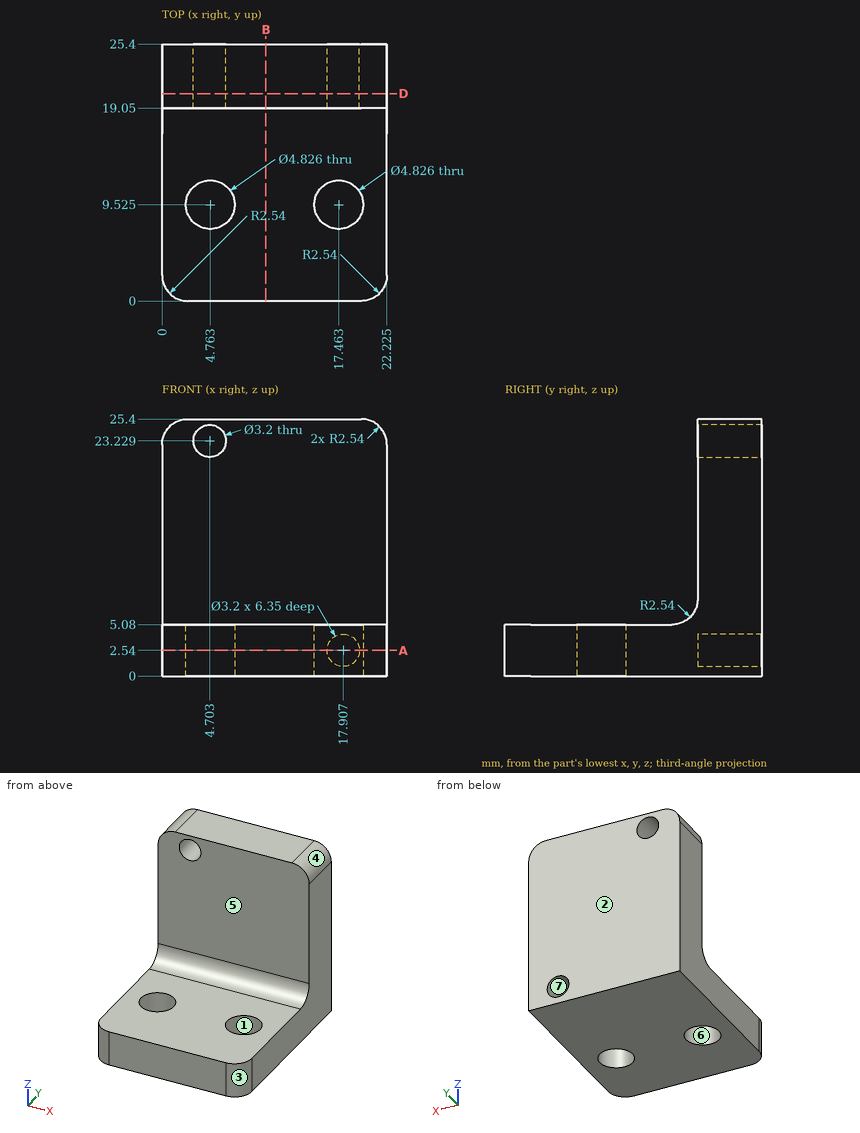
The figure shows three views and two pictorial views of one solid part (mm, origin at its lowest corner). Answer the questions. A direction names the side the tool comes from. Coordinates: 2 decimals unless noted, no trailing zeros. Loops run counter-clockwise (first coordinate to the right, second up) from the corner with the lowest first, then second, coordinate; pieces in that order, holes last. Notation, with made-up numbers: (-34, 13.5) - (1, 13.5) arc R8 ccw to (1, 28.5) - close; hole circle Ø1 at (-22, -7). An arc over 180 degrees is marked (long way). Use a Markdown table: item, result. Add a question column.
1) Find the intervals of material crossed by line 1 (X direction, y = 22.75, z = 2.54) (1 decimal); line 2 (Z direction, x = 20.25, y = 3.5); line 3 (Y direction, x = 7.75, z = 14.75), in increasing order.
2) The mould has two halves that part along Y. Classify the marked faces 1, 2, 3 and 4: released by +Y, released by -Y, zero draft, split by the parting line, or undercut.
3) The part is cut by section D-D, the plane y = 20.5. Give the vertices of the cut face in (x, z) (1 decimal), and give its area (3 significant figures).
4) For the marked faces 5, 6 and 7, determine the directions among +Z, -Z, +X, -X, +Y, -Y from which every point of the face is accessible in a straight line to the end or side of a thin tool.
5) The part is cut by section B-B, the plane x = 10.25. Give the vertices of the cut face in (y, z).
6) Given pin 1 (2.5 mm diameter, centred on x = 17.907, z = 2.54, fed in from +Y); pin 2 (12 mm diameter, centred on x = 8, y = 19.5, fed in from -Z); pin 3 (8 mm diameter, centred on x = 6, z = 15, fed in from -Y); pin 4 (3 mm diameter, centred on x = 4.76, y = 9.52, fed in from -Z), each flat-ended and moving along its own axis, determine where each tip first touches the part or whether it passes through.
7) The part is cut by section A-A, the plane z = 2.54. State how many separate pieces and enclosed holes the cut face has, and give its area (3 significant figures).
Here are the results:
| question | item | result |
|---|---|---|
| 1 | line 1 | x = 0 to 16.3, 19.5 to 22.2 |
| 1 | line 2 | z = 0 to 5.08 |
| 1 | line 3 | y = 19.05 to 25.4 |
| 2 | face 1 | undercut |
| 2 | face 2 | released by +Y |
| 2 | face 3 | released by -Y |
| 2 | face 4 | zero draft |
| 3 | outline | (0, 0) - (22.2, 0) - (22.2, 22.9) arc R2.5 ccw to (19.7, 25.4) - (2.5, 25.4) arc R2.5 ccw to (0, 22.9) - close; hole circle Ø3.2 at (4.7, 23.2); hole circle Ø3.2 at (17.9, 2.5) |
| 3 | area | 546 mm^2 |
| 4 | face 5 | +Z, +X, -X, -Y |
| 4 | face 6 | +Z, -Z |
| 4 | face 7 | +Y |
| 5 | outline | (0, 0) - (25.4, 0) - (25.4, 25.4) - (19.05, 25.4) - (19.05, 7.62) arc R2.54 cw to (16.51, 5.08) - (0, 5.08) - close |
| 6 | pin 1 | stops at y = 19.05 |
| 6 | pin 2 | stops at z = 0 |
| 6 | pin 3 | stops at y = 19.05 |
| 6 | pin 4 | passes through |
| 7 | separate pieces | 1 |
| 7 | enclosed holes | 2 |
| 7 | area | 505 mm^2 |
